Part model, mm, in its own coordinate system. Face numbers are marked on the shaded views. Give positions to 0.01 mm unless a question says otherwise; leave off trailing zeros. Write each loop counter-clockwise with the first axis right and the second up, starting at its lowest first coordinate (ties: lowest second). Pieces come first, ordered by that corner, then holes.
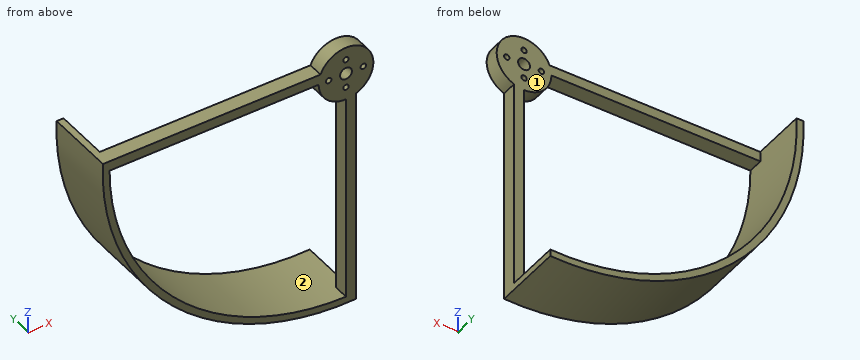
from build123d import *

# Parameters (mm, degrees)
SKETCH1_R           = 15
BOSS_EXTRUDE2_DEPTH = 8.255
BOSS_EXTRUDE3_DEPTH = 8.255
BOSS_EXTRUDE4_DEPTH = 38.1
SKETCH5_R           = 1.500000048
SKETCH5_R_2         = 1.5
SKETCH5_R_3         = 3.249999977
CUT_EXTRUDE3_DEPTH  = 63.5


with BuildPart() as part:
    # Sketch1 → Boss-Extrude2 (new body)
    with BuildSketch(Plane(origin=(0, 0, 0), x_dir=(1, 0, 0), z_dir=(0, 1, 0))):
        Circle(SKETCH1_R)
    extrude(amount=BOSS_EXTRUDE2_DEPTH)

    # Sketch1_6 → Boss-Extrude3 (add)
    with BuildSketch(Plane(origin=(0, 0, 0), x_dir=(1, 0, 0), z_dir=(0, 1, 0))):
        with BuildLine():
            Line((-15, 0), (-129.603225711, 0))
            ThreePointArc((-129.603225711, 0), (-129.574545619, -2.726397307), (-129.488518037, -5.451587957))
            Line((-129.488518037, -5.451587957), (-13.974268809, -5.451587957))
            ThreePointArc((-13.974268809, -5.451587957), (-14.741336984, -2.773622889), (-15, 0))
        make_face()
        with BuildLine():
            ThreePointArc((5.451587957, 129.488518037), (2.726397307, 129.574545619), (0, 129.603225711))
            Line((0, 129.603225711), (0, 15))
            ThreePointArc((0, 15), (2.773622889, 14.741336984), (5.451587957, 13.974268809))
            Line((5.451587957, 13.974268809), (5.451587957, 129.488518037))
        make_face()
    extrude(amount=BOSS_EXTRUDE3_DEPTH)

    # Sketch1_7 → Boss-Extrude4 (add)
    with BuildSketch(Plane(origin=(0, 0, 0), x_dir=(1, 0, 0), z_dir=(0, 1, 0))):
        with BuildLine():
            Line((5.451587957, 129.488518037), (5.451587957, 133.238518037))
            ThreePointArc((5.451587957, 133.238518037), (-94.292689271, 94.292689271), (-133.238518037, -5.451587957))
            Line((-133.238518037, -5.451587957), (-129.488518037, -5.451587957))
            ThreePointArc((-129.488518037, -5.451587957), (-91.643319764, 91.643319764), (5.451587957, 129.488518037))
        make_face()
    extrude(amount=BOSS_EXTRUDE4_DEPTH)

    # Sketch5 → Cut-Extrude3 (cut)
    with BuildSketch(Plane(origin=(0, 8.255, 0), x_dir=(1, 0, 0), z_dir=(0, 1, 0))):
        with Locations((-9.5, 0)):
            Circle(SKETCH5_R)
        with Locations((0, 8)):
            Circle(SKETCH5_R_2)
        with Locations((0, -8)):
            Circle(SKETCH5_R_2)
        with Locations((9.5, 0)):
            Circle(SKETCH5_R)
        Circle(SKETCH5_R_3)
    extrude(amount=-CUT_EXTRUDE3_DEPTH, mode=Mode.SUBTRACT)


solid = part.part
1) Mould opens along Z. For the marked faces 1 and 2 say: +Z half, -Z half, draft (parallel to the pull), parting line (faces both ways), or undercut.
Check result:
face 1: draft
face 2: undercut
2) Saw through at C-C (y = 12). Write the cut outline in (x, z), and give its area (3 significant figures).
Check result:
outline: (-133.24, 5.45) arc R133.35 ccw to (5.45, -133.24) - (5.45, -129.49) arc R129.6 cw to (-129.49, 5.45) - close
area: 815 mm2
3) Saw through at A-A (x = -29.5). Write the cut outline in (y, z) (3 decimals), and give its area (3 significant figures).
Check result:
outline: (0, -130.046) - (38.1, -130.046) - (38.1, -126.201) - (0, -126.201) - close; (0, 0) - (8.255, 0) - (8.255, 5.452) - (0, 5.452) - close
area: 191 mm2
4) Drill centre lines: L1, parallel to X at y = 2, z = -8; L2, parallel to X at y = 3, z = -87; L3, parallel to Y at x = -29.5, z = 1 (3 decimals). Where is each one in solid material? Low to high.
Check result:
L1: x = -133.11 to -129.36, -12.69 to -1.5, 1.5 to 12.69
L2: x = -101.06 to -96.06, 0 to 5.45
L3: y = 0 to 8.255
5) Flat gauge pins, fed straight in: P1, Ø1.8, axis at x = 9.5, z = 0, coming from the -Y side; P2, Ø19, axis at y = 18.5, z = -55, coming from the +X side; P3, Ø4, axis at x = -9.5, z = 0, coming from the +Y side (3 decimals); P4, Ø6, axis at y = 30.5, z = -56, coming from the -X side. Where does each tip first touch, or does it go through?
Check result:
P1: passes through
P2: stops at x = -112.41
P3: stops at y = 8.255
P4: stops at x = -122.37
6) Saw through at B-B (z = -59). Write the cut outline in (x, y) (3 decimals).
Check result:
outline: (-119.588, 0) - (-115.395, 0) - (-115.395, 38.1) - (-119.588, 38.1) - close; (0, 0) - (5.452, 0) - (5.452, 8.255) - (0, 8.255) - close
